Could you check a few things on this model? Use its own coordinates, in mm. Face numbers are marked on the shaded views. Give positions to 0.01 mm unless a question says otherwise; leave off trailing zeros. Write each loop counter-clockwise with the first axis right and the second up, starting at its lowest first coordinate (ties: lowest second). Pieces come first, ordered by that corner, then holes. Notation, with made-up numbers: (26, 32) -> (35, 32) arc R14 ccw to (35, 48) -> close; hole circle Ø9 at (24.5, -23.5). An arc over 180 degrees is marked (long way). Write item = value, one per line. Start each with the question number.
```python
from build123d import *

# Parameters (mm, degrees)
F0_R     = 44
F1_DEPTH = 20
F2_T     = -2
F3_R     = 1
F4_R     = 0.99999
F5_R     = 5


# Not quite as in the source:
# - a fillet or chamfer is up to 0.001 mm smaller than in the source, because OpenCascade refuses the exact size


with BuildPart() as f1:
    # F0 (on Top) → F1 (new body)
    with BuildSketch(Plane.XY):
        Circle(F0_R)
    extrude(amount=F1_DEPTH)

    # F2
    f2_openings = [f1.faces().sort_by_distance(p)[0] for p in [
        (0, 0, 20),
    ]]
    offset(amount=F2_T, openings=f2_openings)

    # F3
    f3_edges = [f1.edges().sort_by_distance(p)[0] for p in [
        (-42, 0, 20),
    ]]
    fillet(f3_edges, radius=F3_R)

    # F4 (radius 1 in the source; OpenCascade refuses exactly that, so slightly less here)
    f4_edges = [f1.edges().sort_by_distance(p)[0] for p in [
        (-44, 0, 20),
    ]]
    fillet(f4_edges, radius=F4_R)

    # F5
    f5_edges = [f1.edges().sort_by_distance(p)[0] for p in [
        (-44, 0, 0),
    ]]
    fillet(f5_edges, radius=F5_R)


solid = f1.part
```
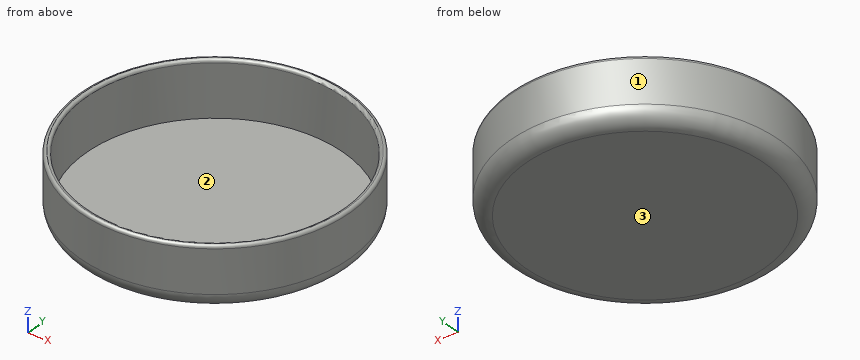
(1) Imagine slicing it at C-C (z = 7.75). Please give me the cut outline in (x, y), then the cut area to 3 significant figures.
(2) If I drill on line 1 along Y through (x, z) = (0, 6.25); line 2 along X through (y, z) = (-4, 12.75); line 3 along X through (y, z) = (21.5, 10.25), over which ranges is the centre line in solid material (lowest first)? Write a range as from..to.
(3) We'd pull the mould along Y, two halves only. Please class the marked faces 1, 2 and 3: released by +Y, released by -Y, zero draft, split by the parting line, or undercut.
(4) I'm going to push flat-ended pins straight in: pin 1 (10 mm diameter, centred on y = -21.5, z = 2, fed in from +X); pin 2 (6 mm diameter, centred on x = -4, z = 12.5, fed in from +Y); pin 3 (10 mm diameter, centred on x = 21, y = -7.5, fed in from +Z). Where does each tip first touch, or does it pass through?
(5) Imagine slicing it at D-D (z = 3.25). Please give me the cut outline in (x, y).
Answers below:
q1.outline = circle Ø88 at (0, 0); hole circle Ø84 at (0, 0)
q1.area = 540 mm^2
q2.line_1 = -44..-42, 42..44
q2.line_2 = -43.82..-41.81, 41.81..43.82
q2.line_3 = -38.39..-36.08, 36.08..38.39
q3.face_1 = split by the parting line
q3.face_2 = undercut
q3.face_3 = zero draft
q4.pin_1 = 40.51
q4.pin_2 = 43.99
q4.pin_3 = 2
q5.outline = circle Ø87.37 at (0, 0); hole circle Ø84 at (0, 0)
